Model file for the job. Use its own axes, mm. A direction names the side the tool comes from. Round coordinates to 2 decimals unless told otherwise and drop trailing zeros. Loops run counter-clockwise (first coordinate to the right, second up) from the corner with the lowest first, then second, coordinate; pieces in that order, holes last.
from build123d import *

# Parameters (mm, degrees)
CYLINDER003_R     = 6
CYLINDER003_DEPTH = 27
CYLINDER002_R     = 2.3
CYLINDER002_DEPTH = 3
ARRAY002_X_COUNT  = 2
ARRAY002_X_PITCH  = 31
ARRAY002_Y_COUNT  = 2
ARRAY002_Y_PITCH  = 75.2
CYLINDER001_R     = 1.3
CYLINDER001_DEPTH = 5
ARRAY001_X_COUNT  = 2
ARRAY001_X_PITCH  = 31
ARRAY001_Y_COUNT  = 2
ARRAY001_Y_PITCH  = 75.2
BOX002_W          = 25
BOX002_H          = 71
BOX002_DEPTH      = 10
CYLINDER_R        = 14
CYLINDER_DEPTH    = 10
ARRAY_Y_COUNT     = 4
ARRAY_Y_PITCH     = 36
BOX001_W          = 100
BOX001_H          = 145
BOX001_DEPTH      = 75
BOX_W             = 105
BOX_H             = 150
BOX_DEPTH         = 78
FILLET_R          = 15
FILLET001_R       = 15
CHAMFER001_SIZE   = 1


with BuildPart() as cilindro003:
    # Cylinder003 → Cylinder003 (new body)
    with BuildSketch(Plane(origin=(10, 9, 51), x_dir=(1, 0, 0), z_dir=(0, 0, 1))):
        Circle(CYLINDER003_R)
    extrude(amount=CYLINDER003_DEPTH)


with BuildPart() as array002:
    # Cylinder002 → Cylinder002 (new body)
    with BuildSketch(Plane(origin=(18, 37.5, 3), x_dir=(1, 0, 0), z_dir=(0, 0, 1))):
        Circle(CYLINDER002_R)
    extrude(amount=CYLINDER002_DEPTH)

    # Array002 X: Array002 ×2


with BuildPart() as array002_1:
    add(array002.part)
    with Locations(*[(i * ARRAY002_X_PITCH, 0, 0) for i in range(1, ARRAY002_X_COUNT)]):
        add(array002.part)

    # Array002 Y: Array002 ×2


with BuildPart() as array002_2:
    add(array002_1.part)
    with Locations(*[(0, i * ARRAY002_Y_PITCH, 0) for i in range(1, ARRAY002_Y_COUNT)]):
        add(array002_1.part)


with BuildPart() as fusion:
    # Cylinder001 → Cylinder001 (new body)
    with BuildSketch(Plane(origin=(18, 37.5, 3), x_dir=(1, 0, 0), z_dir=(0, 0, 1))):
        Circle(CYLINDER001_R)
    extrude(amount=CYLINDER001_DEPTH)

    # Array001 X: Fusion ×2


with BuildPart() as fusion_1:
    add(fusion.part)
    with Locations(*[(i * ARRAY001_X_PITCH, 0, 0) for i in range(1, ARRAY001_X_COUNT)]):
        add(fusion.part)

    # Array001 Y: Fusion ×2


with BuildPart() as fusion_2:
    add(fusion_1.part)
    with Locations(*[(0, i * ARRAY001_Y_PITCH, 0) for i in range(1, ARRAY001_Y_COUNT)]):
        add(fusion_1.part)

    # Fusion: union Array002
    add(array002_2.part)


with BuildPart() as cubo002:
    # Box002 → Box002 (new body)
    with BuildSketch(Plane(origin=(20.5, 39.5, -1), x_dir=(1, 0, 0), z_dir=(0, 0, 1))):
        with Locations((12.5, 35.5)):
            Rectangle(BOX002_W, BOX002_H)
    extrude(amount=BOX002_DEPTH)


with BuildPart() as botones:
    # Cylinder → Cylinder (new body)
    with BuildSketch(Plane(origin=(80, 25, 0), x_dir=(1, 0, 0), z_dir=(0, 0, 1))):
        Circle(CYLINDER_R)
    extrude(amount=CYLINDER_DEPTH)

    # Array Y: Botones ×4


with BuildPart() as botones_1:
    add(botones.part)
    with Locations(*[(0, i * ARRAY_Y_PITCH, 0) for i in range(1, ARRAY_Y_COUNT)]):
        add(botones.part)


with BuildPart() as botones_2:
    # Array placement: moved
    add(botones_1.part.moved(Location((0, -4, -2))))


with BuildPart() as cubo001:
    # Box001 → Box001 (new body)
    with BuildSketch(Plane(origin=(2.5, 2.5, 3), x_dir=(1, 0, 0), z_dir=(0, 0, 1))):
        with Locations((50, 72.5)):
            Rectangle(BOX001_W, BOX001_H)
    extrude(amount=BOX001_DEPTH)


with BuildPart() as chamfer001:
    # Box → Box (new body)
    with BuildSketch(Plane.XY):
        with Locations((52.5, 75)):
            Rectangle(BOX_W, BOX_H)
    extrude(amount=BOX_DEPTH)

    # Cut: cut Cubo001
    add(cubo001.part, mode=Mode.SUBTRACT)

    # Cut001: cut Botones
    add(botones_2.part, mode=Mode.SUBTRACT)

    # Cut002: cut Cubo002
    add(cubo002.part, mode=Mode.SUBTRACT)

    # Fillet
    fillet_edges = [chamfer001.edges().sort_by_distance(p)[0] for p in [
        (2.5, 2.5, 40.5),
        (2.5, 147.5, 40.5),
        (102.5, 2.5, 40.5),
        (102.5, 147.5, 40.5),
    ]]
    fillet(fillet_edges, radius=FILLET_R)

    # Fillet001
    fillet001_edges = [chamfer001.edges().sort_by_distance(p)[0] for p in [
        (0, 0, 39),
        (0, 150, 39),
        (105, 150, 39),
        (105, 0, 39),
    ]]
    fillet(fillet001_edges, radius=FILLET001_R)

    # Fusion001: union Fusion
    add(fusion_2.part)

    # Fusion002: union Cilindro003
    add(cilindro003.part)

    # Chamfer001
    chamfer001_edges = [chamfer001.edges().sort_by_distance(p)[0] for p in [
        (7.575675, 6.252432, 51),
    ]]
    chamfer(chamfer001_edges, length=CHAMFER001_SIZE)


solid = chamfer001.part
Q1. Flat gauge pins, fed straight in: P1, Ø3, axis at x = 64.5, y = 38, coming from the +Z side; P2, Ø3, axis at x = 18.5, y = 37.5, coming from the +Z side; P3, Ø25, axis at x = 80, y = 21, coming from the +Z side. Where does each tip first touch, or does it go through?
Q2. Slice it at B-B on x = 80. Give the cut face in (y, z), plus the area to 3 significant figures.
Q3. Tool access for faces 4 (the face through (52, 0, 38)), 5 (the face through (7.99, 6.86, 50.73)), 6 (the face through (52, 2.5, 40)), 7 (the face through (2, 92, 78)), 8 (the face through (33, 110.5, 1)): list every direction of +Z, -Z, +X, -X, +Y, -Y with a clear straight run to the whole face (end or side of a thin tool).
Q4. Slice it at D-D on y = 57. Give the cut face in (x, z).
Q5. Slice it at C-C on z = 27.5. Give the cut face in (x, y), plus the area to 3 significant figures.
Q6. Slice it at A-A on y = 74. Give the cut face in (x, z), plus the area to 3 significant figures.
Q7. Pull direction X, two halves, no side cores. Call faces 1 (the face through (45.5, 75, 1)), 2 (the face through (0, 74, 38)), 3 (the face through (105, 74, 38)): pulls with the +X half, pulls with the -X half, needs draft (parallel to the pull), parting line crosses it, or undercut.
Q8. Probe line 1 (Y direction, x = 80, z = 1); line 2 (Y direction, x = 74, z = 29.5); line 3 (X direction, y = 93, z = 1.3). List the from-to ranges inside material, lowest first.
Reply:
1. P1: stops at z = 3
1. P2: stops at z = 8
1. P3: passes through
2. outline: (0, 0) - (7, 0) - (7, 3) - (2.5, 3) - (2.5, 78) - (0, 78) - close; (35, 0) - (43, 0) - (43, 3) - (35, 3) - close; (71, 0) - (79, 0) - (79, 3) - (71, 3) - close; (107, 0) - (115, 0) - (115, 3) - (107, 3) - close; (143, 0) - (150, 0) - (150, 78) - (147.5, 78) - (147.5, 3) - (143, 3) - close
2. area: 489 mm2
3. face 4: +Z, -Z, +X, -X, -Y
3. face 5: none
3. face 6: +Z
3. face 7: +Z, +X, -X, +Y, -Y
3. face 8: +Z, -Z
4. outline: (0, 0) - (20.5, 0) - (20.5, 3) - (2.5, 3) - (2.5, 78) - (0, 78) - close; (45.5, 0) - (66, 0) - (66, 3) - (45.5, 3) - close; (94, 0) - (105, 0) - (105, 78) - (102.5, 78) - (102.5, 3) - (94, 3) - close
5. outline: (0, 15) arc R15 ccw to (15, 0) - (90, 0) arc R15 ccw to (105, 15) - (105, 135) arc R15 ccw to (90, 150) - (15, 150) arc R15 ccw to (0, 135) - close; hole (2.5, 17.5) arc R15 ccw to (17.5, 2.5) - (87.5, 2.5) arc R15 ccw to (102.5, 17.5) - (102.5, 132.5) arc R15 ccw to (87.5, 147.5) - (17.5, 147.5) arc R15 ccw to (2.5, 132.5) - close
5. area: 1,250 mm2
6. outline: (0, 0) - (20.5, 0) - (20.5, 3) - (2.5, 3) - (2.5, 78) - (0, 78) - close; (45.5, 0) - (105, 0) - (105, 78) - (102.5, 78) - (102.5, 3) - (45.5, 3) - close
6. area: 615 mm2
7. face 1: undercut
7. face 2: pulls with the -X half
7. face 3: pulls with the +X half
8. line 1: y = 0 to 7, 35 to 43, 71 to 79, 107 to 115, 143 to 150
8. line 2: y = 0 to 2.5, 147.5 to 150
8. line 3: x = 0 to 20.5, 45.5 to 66, 94 to 105
